Read the model definition and answer for the solid it produces. Units are mm, in the model's axes. A direction names the side the tool comes from. Coordinates: 2 decimals unless noted, no trailing zeros. Write each loop counter-clockwise with the first axis right and the second up, starting at its lowest first coordinate (ties: lowest second). Pieces come first, ordered by that corner, then holes.
(1) Which of the six approach directions +Z, -Z, +X, -X, +Y, -Y give full straight-line access (tool end or side, diameter ignored) to faces 1 (the flat face through (-8, 14, 5)), 2 (the cylindrical face through (3.884, -9.755, 4.93)), 3 (the flat face through (-10, 12, 5))?
(2) Section C-C on x = 7 is taken. Write down the section's boundary in (y, z).
(3) Section A-A on y = 0 is taken. Write down the section's boundary in (x, z).
(4) Find the intervals of material crossed by probe 1 along Y at (x, z) = (7, 8.5); probe 2 along X at (y, z) = (3, 2); probe 3 along Y at (x, z) = (-2, 6.75), in increasing order.
(5) Section B-B on z = 3.5 is taken. Write down the section's boundary in (x, y), then the cut area to 3 significant figures.
(6) Given pin 1 (3 mm diameter, centred on y = 8.5, z = 1.5, fed in from -X); pin 2 (1 mm diameter, centred on x = 1, z = 6, fed in from -Y); pin 3 (4.5 mm diameter, centred on y = 14.5, z = 4.5, fed in from +X); pin 4 (3 mm diameter, centred on x = -2.5, y = 9.5, fed in from +Z), each flat-ended and moving along its own axis, determine where each tip first touches the part or whether it passes through.
(7) The mould has two halves that part along X. Classify faces 4 (the flat face through (0, 14, 5)), 5 (the flat face through (-9, 16.455, 5)), 6 (the cylindrical face through (3.104, 12.052, 4.93)), 7 (the cylindrical face through (-2.17, -9.76, 4.93)): +X half, -X half, draft (parallel to the pull), parting line (faces both ways), or undercut.
from build123d import *

# Parameters (mm, degrees)
SKETCH1_R           = 10.5
SKETCH1_R_2         = 10
BOSS_EXTRUDE1_DEPTH = 10
FILLET1_R           = 50
FILLET2_R           = 10


with BuildPart() as part:
    # Sketch1 → Boss-Extrude1 (new body)
    # profile 1 of 2: a face of its own
    with BuildSketch(Plane.XY):
        with BuildLine():
            Line((-8, 16.455448816), (-10, 16.455448816))
            Line((-10, 16.455448816), (-10, 3.201562119))
            ThreePointArc((-10, 3.201562119), (-5.350189391, 9.034681703), (2, 10.307764064))
            Line((2, 10.307764064), (2, 16.455448816))
            Line((2, 16.455448816), (0, 16.455448816))
            Line((0, 16.455448816), (0, 12.455448816))
            Line((0, 12.455448816), (-8, 12.455448816))
            Line((-8, 12.455448816), (-8, 16.455448816))
        make_face()
    # profile 2 of 2: a face of its own
    with BuildSketch(Plane.XY):
        Circle(SKETCH1_R)
        Circle(SKETCH1_R_2, mode=Mode.SUBTRACT)
    extrude(amount=BOSS_EXTRUDE1_DEPTH)

    # Fillet1
    fillet1_edges = [part.edges().sort_by_distance(p)[0] for p in [
        (-10, 3.201562119, 5),
    ]]
    fillet(fillet1_edges, radius=FILLET1_R)

    # Fillet2
    # the kernel refuses this fillet: 10 mm, written as the material it adds along each edge
    with BuildSketch(Plane(origin=(2, 10.307764064, 0), x_dir=(0.9177385180752605, -0.3971851110515409, 0), z_dir=(0, 0, 1))) as fillet2_piece_1:
        with BuildLine():
            CenterArc((6.668287117, 9.765906989), FILLET2_R, 204.355310462, 53.22294126)
            Line((-2.441768851, 5.641967094), (-2.62396997, 5.559488296))
            ThreePointArc((-2.62396997, 5.559488296), (-1.404432129, 2.741546525), (-0.183547704, -0.079437022))
            Line((-0.183547704, -0.079437022), (0.043021207, -0.19531814))
            ThreePointArc((0.043021207, -0.19531814), (2.258613378, 0.045797661), (4.474205549, -0.19531814))
            Line((4.474205549, -0.19531814), (4.517226757, 0))
        make_face()
    extrude(amount=10)


solid = part.part
Response:
1. face 1: +Z, -Z, +Y
1. face 2: +Z, -Z
1. face 3: +Z, -Z, -X, +Y
2. outline: (-7.83, 0) - (-7.14, 0) - (-7.14, 10) - (-7.83, 10) - close; (7.14, 0) - (7.83, 0) - (7.83, 10) - (7.14, 10) - close
3. outline: (-10.5, 0) - (-10, 0) - (-10, 10) - (-10.5, 10) - close; (10, 0) - (10.5, 0) - (10.5, 10) - (10, 10) - close
4. probe 1: y = -7.83 to -7.14, 7.14 to 7.83
4. probe 2: x = -10.23 to -9.54, 9.54 to 10.06
4. probe 3: y = -10.31 to -9.8, 9.8 to 12.46
5. outline: (-10.41, 1.35) arc R10.5 ccw (long way) to (6.15, 8.51) arc R10 cw to (2, 16.46) - (0, 16.46) - (0, 12.46) - (-8, 12.46) - (-8, 16.46) - (-10, 16.46) - (-10, 7.76) arc R50 cw to start; hole circle Ø20 at (0, 0)
5. area: 97.3 mm2
6. pin 1: stops at x = -10.01
6. pin 2: stops at y = -10.49
6. pin 3: stops at x = 3
6. pin 4: stops at z = 10
7. face 4: undercut
7. face 5: draft
7. face 6: +X half
7. face 7: undercut
